Input: part model. Units: mm. Frame: model coordinates. Face numbers are marked on the shaded views. A direction names the side the tool comes from. Round coordinates to 2 decimals unless told otherwise and drop trailing zeros. Loops run counter-clockwise (first coordinate to the right, second up) from the corner with the lowest first, then second, coordinate; pieces in that order, holes last. Notation, with made-up numbers: (4, 1.25) -> (21, 1.25) arc R33 cw to (21, 33.25) -> close; hole circle Ø7 at (8.5, 28). An arc over 180 degrees is marked (long way). Answer as a JSON object with one key per item and string values.
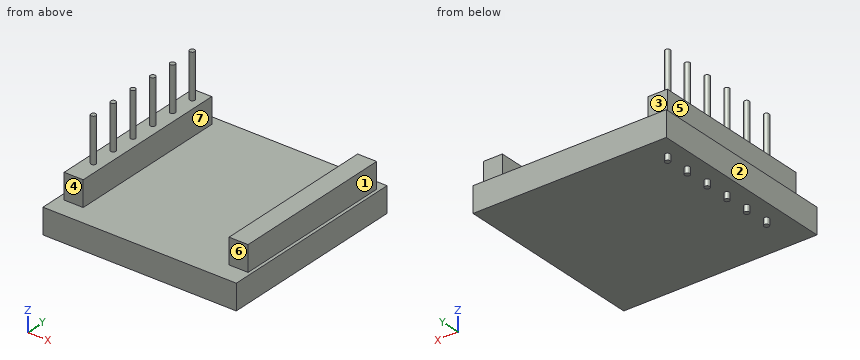
```python
from build123d import *

# Parameters (mm, degrees)
SKETCH_1_W           = 15.24
SKETCH_1_H           = 15.24
EXTRUDE_1_DEPTH      = 2
SKETCH_2_W           = 1.5
SKETCH_2_H           = 13
EXTRUDE_2_DEPTH      = 2
EXTRUDE_3_DEPTH      = 3.5
EXTRUDE_3_DEPTH_BACK = 4.5
SKETCH_3_R           = 0.2


with BuildPart() as part:
    # 草图1 → 凸台-拉伸1 (new body)
    with BuildSketch(Plane.XY):
        with Locations((7.62, 7.62)):
            Rectangle(SKETCH_1_W, SKETCH_1_H)
    extrude(amount=EXTRUDE_1_DEPTH)

    # 草图2 → 凸台-拉伸2 (add)
    with BuildSketch(Plane.XY.offset(2)):
        with Locations((14.25, 8)):
            Rectangle(SKETCH_2_W, SKETCH_2_H)
        with Locations((1.25, 8)):
            Rectangle(SKETCH_2_W, SKETCH_2_H)
    extrude(amount=EXTRUDE_2_DEPTH)

    # 草图3 → 凸台-拉伸3 (add, two sides: drawn at the far end of the back side and taken through both)
    with BuildSketch(Plane.XY.offset(4).offset(-EXTRUDE_3_DEPTH_BACK)):
        with Locations((1.25, 13.5)):
            Circle(SKETCH_3_R)
        with Locations((1.25, 11.5)):
            Circle(SKETCH_3_R)
        with Locations((1.25, 9.5)):
            Circle(SKETCH_3_R)
        with Locations((1.25, 7.5)):
            Circle(SKETCH_3_R)
        with Locations((1.25, 5.5)):
            Circle(SKETCH_3_R)
        with Locations((1.25, 3.5)):
            Circle(SKETCH_3_R)
    extrude(amount=EXTRUDE_3_DEPTH + EXTRUDE_3_DEPTH_BACK)


solid = part.part
```
1) Reachability of the marked faces 1, 2, 3 and 4 from +Z, -Z, +X, -X, +Y, -Y: full face, straight path, thin tool, end or side. Return the list, or none.
Output:
{"face 1": "+Z, +X, +Y, -Y", "face 2": "+Z, -Z, -X, +Y, -Y", "face 3": "+Z, +X, -X, +Y", "face 4": "+Z, +X, -X, -Y"}
2) Section B-B, the plane x = 8. Output: boundary loops of the cut face in (y, z), plus the area to 3 significant figures.
Output:
{"outline": "(0, 0) -> (15.24, 0) -> (15.24, 2) -> (0, 2) -> close", "area": "30.5 mm^2"}
3) Section A-A, the plane y = 2.5. Output: boundary loops of the cut face in (x, z), plus the area to 3 significant figures.
Output:
{"outline": "(0, 0) -> (15.24, 0) -> (15.24, 2) -> (15, 2) -> (15, 4) -> (13.5, 4) -> (13.5, 2) -> (2, 2) -> (2, 4) -> (0.5, 4) -> (0.5, 2) -> (0, 2) -> close", "area": "36.5 mm^2"}
4) Ray query, probe 1 along Y at (x, z) = (1.25, 5.5); probe 2 along X at (y, z) = (9.25, 2.25); probe 3 along Z at (x, y) = (7.75, 12.25). Return the intervals inside material, ascending.
Output:
{"probe 1": "y = 3.3 to 3.7, 5.3 to 5.7, 7.3 to 7.7, 9.3 to 9.7, 11.3 to 11.7, 13.3 to 13.7", "probe 2": "x = 0.5 to 2, 13.5 to 15", "probe 3": "z = 0 to 2"}
5) Contact query for flat-ended pins moving along their axis: P1, Ø0.6, axis at y = 9.5, z = 3, coming from the +X side; P2, Ø1.2, axis at x = 14.5, z = 3, coming from the +Y side; P3, Ø1.2, axis at x = 14.5, z = 3.5, coming from the -Y side. Output: stop coordinate, or through.
Output:
{"P1": "stops at x = 15", "P2": "stops at y = 14.5", "P3": "stops at y = 1.5"}
6) Draft query along X for the marked faces 5, 6 and 7. Return one class per face: +X half, -X half, draft (parallel to the pull), parting line (faces both ways), or undercut.
Output:
{"face 5": "-X half", "face 6": "draft", "face 7": "undercut"}
